from build123d import *

# Parameters (mm, degrees)
SKETCH_1_W          = 80
SKETCH_1_H          = 60
EXTRUDE_1_DEPTH     = 2
SKETCH_2_W          = 80
SKETCH_2_H          = 60
SKETCH_2_W_2        = 78
SKETCH_2_H_2        = 58
EXTRUDE_2_DEPTH     = 20
CHAMFER_1_SIZE      = 1
SKETCH_3_W          = 12.489594438
SKETCH_3_H          = 12.7
SKETCH_3_W_2        = 12.168468818
SKETCH_3_H_2        = 9.816130436
CUT_EXTRUDE_1_DEPTH = 10
SKETCH_4_R          = 3.431381937
SKETCH_4_R_2        = 2
SKETCH_4_R_3        = 3.312453099
SKETCH_4_R_4        = 3.867665241
SKETCH_4_R_5        = 3.660588401
EXTRUDE_4_DEPTH     = 4
CHAMFER_2_SIZE      = 0.4


with BuildPart() as part:
    # Эскиз1 → Бобышка-Вытянуть1 (new body)
    with BuildSketch(Plane.XY):
        with Locations((18.021978022, -0.32967033)):
            Rectangle(SKETCH_1_W, SKETCH_1_H)
    extrude(amount=EXTRUDE_1_DEPTH)

    # Эскиз2 → Бобышка-Вытянуть2 (add)
    with BuildSketch(Plane.XY.offset(2)):
        with Locations((18.021978022, -0.32967033)):
            Rectangle(SKETCH_2_W, SKETCH_2_H)
        with Locations((18.021978022, -0.32967033)):
            Rectangle(SKETCH_2_W_2, SKETCH_2_H_2, mode=Mode.SUBTRACT)
    extrude(amount=EXTRUDE_2_DEPTH)

    # Фаска1
    chamfer_1_edges = [part.edges().sort_by_distance(p)[0] for p in [
        (18.021978022, 29.67032967, 0),
        (58.021978022, -0.32967033, 0),
        (18.021978022, -30.32967033, 0),
        (-21.978021978, -0.32967033, 0),
    ]]
    chamfer(chamfer_1_edges, length=CHAMFER_1_SIZE)

    # Эскиз3 → Вырез-Вытянуть1 (cut)
    with BuildSketch(Plane.ZY.offset(21.978021978)):
        with Locations((13.484797219, 13.07032967)):
            Rectangle(SKETCH_3_W, SKETCH_3_H)
        with Locations((13.033283453, -16.331339337)):
            Rectangle(SKETCH_3_W_2, SKETCH_3_H_2)
    extrude(amount=-CUT_EXTRUDE_1_DEPTH, mode=Mode.SUBTRACT)

    # Эскиз4 → Бобышка-Вытянуть4 (add)
    # profile 1 of 4: a face of its own
    with BuildSketch(Plane.XY.offset(2)):
        with Locations((-5.749056018, 26.121666888)):
            Circle(SKETCH_4_R)
        with Locations((-5.749056018, 26.121666888)):
            Circle(SKETCH_4_R_2, mode=Mode.SUBTRACT)
    # profile 2 of 4: a face of its own
    with BuildSketch(Plane.XY.offset(2)):
        with Locations((45.270920547, 10.86273616)):
            Circle(SKETCH_4_R_3)
        with Locations((45.270920547, 10.86273616)):
            Circle(SKETCH_4_R_2, mode=Mode.SUBTRACT)
    # profile 3 of 4: a face of its own
    with BuildSketch(Plane.XY.offset(2)):
        with Locations((45.285382916, -17.058588577)):
            Circle(SKETCH_4_R_4)
        with Locations((45.285382916, -17.058588577)):
            Circle(SKETCH_4_R_2, mode=Mode.SUBTRACT)
    # profile 4 of 4: a face of its own
    with BuildSketch(Plane.XY.offset(2)):
        with Locations((-5.732841378, -22.138175863)):
            Circle(SKETCH_4_R_5)
        with Locations((-5.732841378, -22.138175863)):
            Circle(SKETCH_4_R_2, mode=Mode.SUBTRACT)
    extrude(amount=EXTRUDE_4_DEPTH)

    # Фаска2
    chamfer_2_edges = [part.edges().sort_by_distance(p)[0] for p in [
        (18.021978022, 28.67032967, 22),
        (-20.978021978, -0.32967033, 22),
        (18.021978022, -29.32967033, 22),
        (57.021978022, -0.32967033, 22),
    ]]
    chamfer(chamfer_2_edges, length=CHAMFER_2_SIZE)


solid = part.part
The model under review builds one solid part; all positions refer to its coordinate system, in mm. Give positions to 0.01 mm unless a question says otherwise; leave off trailing zeros. Write each loop counter-clockwise with the first axis right and the second up, starting at its lowest first coordinate (ties: lowest second). Pieces come first, ordered by that corner, then holes.
1. Draft analysis for pull direction X (two halves, no side actions). For faces 1 (the cylindrical face through (-6.17, -24.09, 3.97)), 2 (the flat face through (-21.978, -1, 11)), state which applies: +X half, -X half, draft (parallel to the pull), parting line (faces both ways), or undercut.
2. For P1, Ø8, axis at x = -6, y = -20.5, coming from the +Z side; P2, Ø4, axis at x = 30.5, y = 14.5, coming from the +Z side, all flat-tipped, find the tip position at first contact; note any pin that passes through.
3. Wall thickness on L1, parallel to Y at x = 20, z = 4.75; L2, parallel to X at y = 9.5, z = 20.25; L3, parallel to X at y = 18, z = 14: over which ranges is each line inside the solid? List them lowest first.
4. Add section D-D, the plane x = 35. Write out the cut boundary in (y, z).
5. Add section C-C, the plane z = 4. Count the separate pieces of the cut face and the enclosed holes in it, plus the area to 3 significant figures.
6. Add section B-B, the plane y = 15. Write out the cut boundary in (x, z).
7. Add section A-A, the plane z = 17.5. Write out the cut boundary in (x, y).
Worked answers:
1. face 1: undercut
1. face 2: -X half
2. P1: stops at z = 6
2. P2: stops at z = 2
3. L1: y = -30.33 to -29.33, 28.67 to 29.67
3. L2: x = -21.98 to -20.98, 57.02 to 58.02
3. L3: x = 57.02 to 58.02
4. outline: (-30.33, 1) - (-29.33, 0) - (28.67, 0) - (29.67, 1) - (29.67, 22) - (29.07, 22) - (28.67, 21.6) - (28.67, 2) - (-29.33, 2) - (-29.33, 21.6) - (-29.73, 22) - (-30.33, 22) - close
5. separate pieces: 4
5. enclosed holes: 5
5. area: 384 mm2
6. outline: (-21.98, 1) - (-20.98, 0) - (57.02, 0) - (58.02, 1) - (58.02, 22) - (57.42, 22) - (57.02, 21.6) - (57.02, 2) - (-20.98, 2) - (-20.98, 7.24) - (-21.98, 7.24) - close; (-21.98, 19.73) - (-20.98, 19.73) - (-20.98, 21.6) - (-21.38, 22) - (-21.98, 22) - close
7. outline: (-21.98, -30.33) - (58.02, -30.33) - (58.02, 29.67) - (-21.98, 29.67) - (-21.98, 19.42) - (-20.98, 19.42) - (-20.98, 28.67) - (57.02, 28.67) - (57.02, -29.33) - (-20.98, -29.33) - (-20.98, -21.24) - (-21.98, -21.24) - close; (-21.98, -11.42) - (-20.98, -11.42) - (-20.98, 6.72) - (-21.98, 6.72) - close
